Check sheet for the modelled part. Datum: model origin and axes. Units: mm. A direction names the side the tool comes from. Coordinates: 2 decimals unless noted, no trailing zeros. Write each loop counter-clockwise with the first axis right and the second up, starting at its lowest first coordinate (ties: lowest second). Pieces come first, ordered by that corner, then holes. Notation, with made-up numbers: M 46.25,59 L 98.25,59 A21 cw 98.25,94 Z; hole C 63.5,27.5 d3. An arc over 180 degrees is marked long. Answer as CSV lines item,"result". Start each with the question number.
Q1. Sectioned sample at A-A, the plane x = 2.5. Record the cut outline in (y, z), then the cut area to 3 significant figures.
Q2. Sectioned sample at B-B, the plane z = -15. Record the cut outline in (x, y).
Q3. Mould release check, pull along X, two halves, no side actions. Record for faces 1 (the cylindrical face through (20, 3, -15)), 2 (the flat face through (3, 3, -30)), 3 (the cylindrical face through (5.804, 4.378, -4.508)): pulls with the +X half, pulls with the -X half, needs draft (parallel to the pull), parting line crosses it, or undercut.
Q4. Thickness scan on line 1 along X through (y, z) = (2.75, -15); line 2 along X through (y, z) = (0.9, -15); line 3 along Y through (x, z) = (0.5, -20.5). Record the ranges inside material, lowest first. Write a range as from..to.
Q5. Depth check by flat-ended pin: pin 1 Ø13 at (x, z) = (2.5, -15) entering from -Y; pin 2 Ø1.5 at (y, z) = (4.5, -16) entering from -X; pin 3 Ø3 at (x, z) = (-6, -18) entering from +Y. Enter the tip coordinate at first touch or a pass-through.
Q6. Access from +Z, -Z, +X, -X, +Y, -Y to the whole of each face (thin tool, end or side, straight path). Record for faces 4 (the flat face through (-2, 0, -19)), 5 (the flat face through (0, 2.35, -10)).
Q7. Sectioned sample at D-D, the plane z = -18.5. Record the cut outline in (x, y).
Q8. Sectioned sample at C-C, the plane y = 4.25. Record the cut outline in (x, z).
from build123d import *

# Parameters (mm, degrees)
SKETCH3_R            = 5
BOSS_EXTRUDE1_DEPTH  = 6.35
SKETCH4_R            = 11
CUT_EXTRUDE1_DEPTH   = 4
M3_CLEARANCE_HOLE1_D = 3.4


with BuildPart() as part:
    # Sketch3 → Boss-Extrude1 (new body)
    with BuildSketch(Plane(origin=(0, 0, 0), x_dir=(1, 0, 0), z_dir=(0, 1, 0))):
        with BuildLine():
            Line((0, 0), (5, 0))
            ThreePointArc((5, 0), (20, 15), (5, 30))
            Line((5, 30), (0, 30))
            ThreePointArc((0, 30), (-15, 15), (0, 0))
        make_face()
        with Locations(Location((2.5, 15, 0), (0, 0, 270))):
            Circle(SKETCH3_R, mode=Mode.SUBTRACT)
    extrude(amount=BOSS_EXTRUDE1_DEPTH)

    # Sketch4 → Cut-Extrude1 (cut)
    with BuildSketch(Plane(origin=(0, 6.35, 0), x_dir=(1, 0, 0), z_dir=(0, 1, 0))):
        with Locations(Location((2.5, 15, 0), (0, 0, 270))):
            Circle(SKETCH4_R)
    extrude(amount=-CUT_EXTRUDE1_DEPTH, mode=Mode.SUBTRACT)

    # M3 Clearance Hole1 (through all)
    with Locations(Plane(origin=(-12.5, 6.35, -15), x_dir=(0, 0, 1), z_dir=(0, 1, 0))):
        with Locations((0, 0), (0, 30)):
            Hole(M3_CLEARANCE_HOLE1_D / 2)


solid = part.part
Output:
1,outline,"M 0,-30 L 6.35,-30 L 6.35,-26 L 2.35,-26 L 2.35,-20 L 0,-20 Z; M 0,-10 L 2.35,-10 L 2.35,-4 L 6.35,-4 L 6.35,0 L 0,0 Z"
1,area,"79.0 mm^2"
2,outline,"M -15,0 L -14.2,0 L -14.2,6.35 L -15,6.35 Z; M -10.8,0 L -2.5,0 L -2.5,2.35 L -8.5,2.35 L -8.5,6.35 L -10.8,6.35 Z; M 7.5,0 L 15.8,0 L 15.8,6.35 L 13.5,6.35 L 13.5,2.35 L 7.5,2.35 Z; M 19.2,0 L 20,0 L 20,6.35 L 19.2,6.35 Z"
3,face 1,"pulls with the +X half"
3,face 2,"needs draft"
3,face 3,"undercut"
4,line 1,"x = -15..-14.2, -10.8..-8.5, 13.5..15.8, 19.2..20"
4,line 2,"x = -15..-14.2, -10.8..-2.5, 7.5..15.8, 19.2..20"
4,line 3,"y = 0..2.35"
5,pin 1,"stops at y = 0"
5,pin 2,"stops at x = -15"
5,pin 3,"stops at y = 2.35"
6,face 4,"+Z, -Z, +X, -X, -Y"
6,face 5,"+Y"
7,outline,"M -14.59,0 L -1.07,0 L -1.07,2.35 L -7.93,2.35 L -7.93,6.35 L -14.59,6.35 Z; M 6.07,0 L 19.59,0 L 19.59,6.35 L 12.93,6.35 L 12.93,2.35 L 6.07,2.35 Z"
8,outline,"M 0,-30 L 5,-30 A15 ccw 5,0 L 0,0 A15 ccw Z; hole C -12.5,-15 d3.4; hole C 2.5,-15 d22; hole C 17.5,-15 d3.4"
